The figure shows three views and two pictorial views of one solid part (mm, origin at its lowest corner). Answer the questions. Give positions to 0.01 mm unless a question says otherwise; leave off trailing zeros. Loops run counter-clockwise (first coordinate to the right, second up) from the corner with the lowest first, then second, coordinate; pieces in that order, holes last. Notation, with made-up numbers: M 16.5,20.5 L 53.5,20.5 A26 ccw 53.5,51.5 Z; hole C -15.5,50.5 d9. An arc over 180 degrees is marked long. Answer in a Markdown table with one row per item. Add a question column.
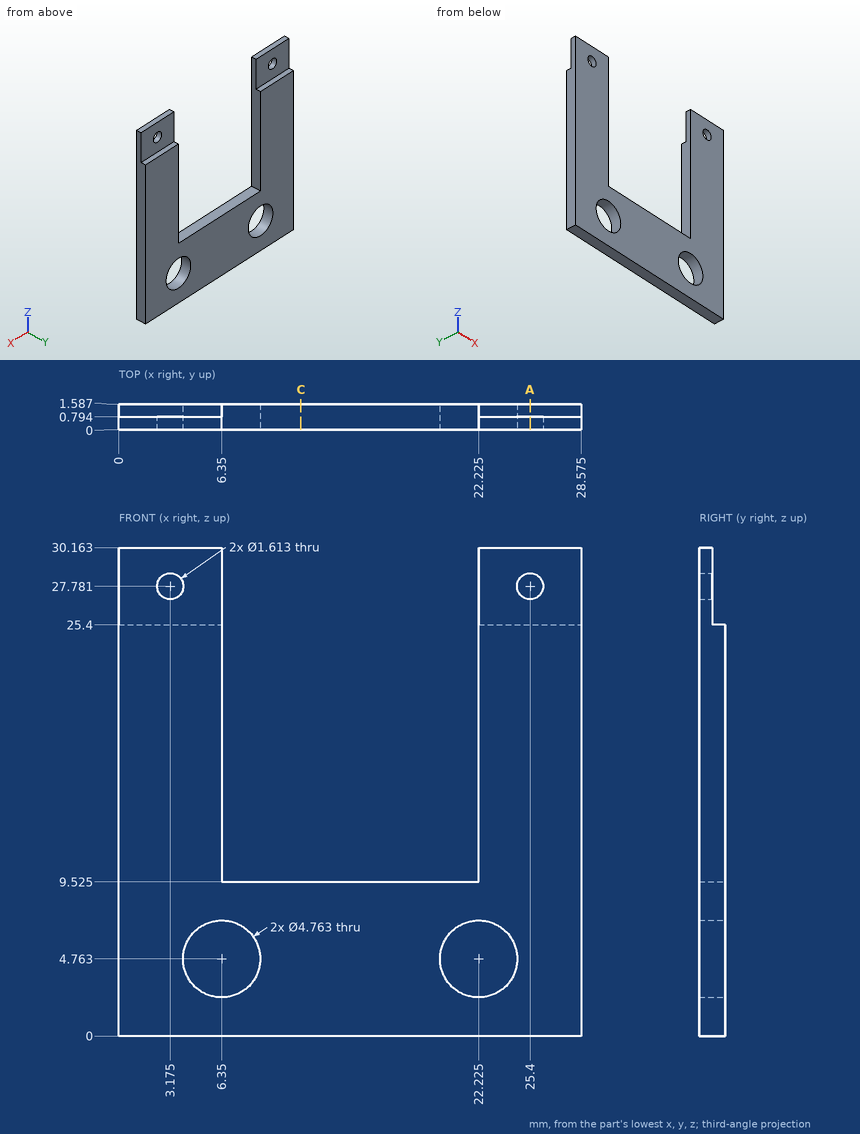
(1) Each of these flat-tipped pins is pushed along its axis until it touches: P1, Ø1.5, axis at x = 21, z = 25.5, coming from the -Y side; P2, Ø1.9, axis at x = 3.18, z = 27.78, coming from the +Y side; P3, Ø0.5, axis at x = 12, y = 0.5, coming from the +Z side (1 decimal). Where does it stop, or does it pass through?
(2) Section A-A, the plane x = 25.4 is taken. Determine the outline of the cut face in (y, z) (1 decimal).
(3) Section C-C, the plane x = 11.25 is taken. Determine the outline of the cut face in (y, z) (1 decimal).
(4) Consider line 1 along Z through (x, y) = (25.4, 0.3) (1 decimal); line 2 along Z through (x, y) = (17, 0.1) (1 decimal); line 3 along Z through (x, y) = (21.25, 0.15) (1 decimal). Determine where each line is inside the solid, lowest interval first. Write a range as from..to.
Numbers:
| question | item | result |
|---|---|---|
| 1 | P1 | passes through |
| 1 | P2 | stops at y = 0.79 |
| 1 | P3 | stops at z = 9.5 |
| 2 | outline | M 0,0 L 1.6,0 L 1.6,25.4 L 0.8,25.4 L 0.8,27 L 0,27 Z; M 0,28.6 L 0.8,28.6 L 0.8,30.2 L 0,30.2 Z |
| 3 | outline | M 0,0 L 1.6,0 L 1.6,9.5 L 0,9.5 Z |
| 4 | line 1 | z = 0..27, 28.6..30.2 |
| 4 | line 2 | z = 0..9.5 |
| 4 | line 3 | z = 0..2.6, 6.9..9.5 |
